from build123d import *

# Parameters (mm, degrees)
CROQUIS1_W              = 150
CROQUIS1_H              = 150
SALIENTE_EXTRUIR1_DEPTH = 10
CROQUIS2_R              = 40
SALIENTE_EXTRUIR2_DEPTH = 40
CORTAR_EXTRUIR1_DEPTH   = 41
CROQUIS4_W              = 20
CROQUIS4_H              = 7.5
CORTAR_EXTRUIR2_DEPTH   = 11.5
CORTAR_EXTRUIR3_START   = -27
CROQUIS5_W              = 20
CROQUIS5_H              = 34.531245334
CORTAR_EXTRUIR3_DEPTH   = 13


with BuildPart() as part:
    # Croquis1 → Saliente-Extruir1 (new body)
    with BuildSketch(Plane(origin=(0, 0, 0), x_dir=(0, 1, 0), z_dir=(0, 0, 1))):
        Rectangle(CROQUIS1_W, CROQUIS1_H)
    extrude(amount=SALIENTE_EXTRUIR1_DEPTH)

    # Croquis2 → Saliente-Extruir2 (add)
    with BuildSketch(Plane.XY.offset(10)):
        Circle(CROQUIS2_R)
    extrude(amount=SALIENTE_EXTRUIR2_DEPTH)

    # Croquis3 → Cortar-Extruir1 (cut)
    with BuildSketch(Plane.XY.offset(50)):
        Polygon((0, 10), (-10, 10), (-10, -30.6), (10, -30.6), (10, 10), align=None)
    extrude(amount=-CORTAR_EXTRUIR1_DEPTH, mode=Mode.SUBTRACT)

    # Croquis4 → Cortar-Extruir2 (cut)
    with BuildSketch(Plane.XY.offset(50)):
        with Locations((0, -34.35)):
            Rectangle(CROQUIS4_W, CROQUIS4_H)
        with Locations((0, 13.75)):
            Rectangle(CROQUIS4_W, CROQUIS4_H)
    extrude(amount=-CORTAR_EXTRUIR2_DEPTH, mode=Mode.SUBTRACT)

    # Croquis5 → Cortar-Extruir3 (cut)
    with BuildSketch(Plane.XY.offset(50).offset(CORTAR_EXTRUIR3_START)):
        with Locations((0, 27.265622667)):
            Rectangle(CROQUIS5_W, CROQUIS5_H)
    extrude(amount=-CORTAR_EXTRUIR3_DEPTH, mode=Mode.SUBTRACT)


solid = part.part
Source: CAD feature listing. Evaluate the final solid. Frame: model axes, mm. A direction names the side the tool comes from. Give positions to 0.01 mm unless a question says otherwise; leave off trailing zeros. Write each loop counter-clockwise with the first axis right and the second up, starting at its lowest first coordinate (ties: lowest second). Pieces come first, ordered by that corner, then holes. Notation, with made-up numbers: (11, 50) -> (67, 50) arc R20 ccw to (67, 73) -> close; hole circle Ø7 at (82.5, 2.25). An arc over 180 degrees is marked (long way). Write item = value, one per line.
Q1. First-contact query: pin 1 (10 mm diameter, centred on y = 14, z = 34.5, fed in from +X); pin 2 (17 mm diameter, centred on x = 4, z = 32, fed in from -Y); pin 3 (20.5 mm diameter, centred on y = 13.5, z = 28, fed in from -X); pin 4 (1.5 mm diameter, centred on y = -42, z = 40, fed in from +X). Flat tips, straight axial feed; report the tip coordinate or a pass-through.
Here are the results:
pin_1 = 38.97
pin_2 = -40
pin_3 = -39.87
pin_4 = through
Q2. Cut plane D-D on y = 0. Return loops of the section in (x, z), then the cut area to 3 significant figures.
Here are the results:
outline = (-75, 0) -> (75, 0) -> (75, 10) -> (40, 10) -> (40, 50) -> (10, 50) -> (10, 9) -> (-10, 9) -> (-10, 50) -> (-40, 50) -> (-40, 10) -> (-75, 10) -> close
area = 3,880 mm²
Q3. Line query: line 1 (Z direction, x = 0.5, y = 17); line 2 (X direction, y = -1, z = 32); line 3 (Z direction, x = -48.5, y = -15). Output: solid intervals per line, ascending. Write a range as from..to.
Here are the results:
line_1 = 0..10, 23..38.5
line_2 = -39.99..-10, 10..39.99
line_3 = 0..10
Q4. Cut plane B-B on x = 0. Return loops of the section in (y, z), then the cut area to 3 significant figures.
Here are the results:
outline = (-75, 0) -> (75, 0) -> (75, 10) -> (10, 10) -> (10, 9) -> (-30.6, 9) -> (-30.6, 38.5) -> (-38.1, 38.5) -> (-38.1, 50) -> (-40, 50) -> (-40, 10) -> (-75, 10) -> close; (10, 23) -> (40, 23) -> (40, 50) -> (17.5, 50) -> (17.5, 38.5) -> (10, 38.5) -> close
area = 2,470 mm²
Q5. Cut plane A-A on y = 32. Return loops of the section in (x, z), then the cut area to 3 significant figures.
Here are the results:
outline = (-75, 0) -> (75, 0) -> (75, 10) -> (24, 10) -> (24, 50) -> (-24, 50) -> (-24, 10) -> (-75, 10) -> close; hole (-10, 10) -> (10, 10) -> (10, 23) -> (-10, 23) -> close
area = 3,160 mm²
Q6. Reachability of faces 5 (the face through (-10, 0, 30)), 6 (the face through (0, -30.6, 24)), 7 (the face through (-1, 18, 50)) from +Z, -Z, +X, -X, +Y, -Y: full face, straight path, thin tool, end or side. Return the list, or none.
Here are the results:
face_5 = none
face_6 = +Z
face_7 = +Z, +X, -X, +Y, -Y
Q7. Mould query, pull axis Z, two halves, no side actions, for faces 1 (the face through (0, -10, 9)), 2 (the face through (75, -1, 5)), 3 (the face through (0, 25, 23)), 4 (the face through (10, 0, 30)). Classes: +Z half, -Z half, draft (parallel to the pull), parting line (faces both ways), or undercut.
Here are the results:
face_1 = +Z half
face_2 = draft
face_3 = undercut
face_4 = undercut
Q8. Cut plane C-C on z = 31. Return loops of the section in (x, y), then the cut area to 3 significant figures.
Here are the results:
outline = circle Ø80 at (0, 0); hole (-10, -30.6) -> (10, -30.6) -> (10, 10) -> (-10, 10) -> close
area = 4,210 mm²
